Work out the finished part from the listing and answer in its coordinate system (mm). A direction names the side the tool comes from. Round coordinates to 2 decimals unless told otherwise and drop trailing zeros. Order: outer loops, then holes, each group sorted by start corner. A loop starts at its lowest first (then second) coordinate and runs counter-clockwise, first axis right, second up. Notation, with made-up numbers: (-26, 68.25) - (3, 68.25) arc R22 ccw to (3, 80.25) - close; hole circle Ø3 at (88, 35). An arc over 180 degrees is marked (long way). Answer in a Markdown table with one row per item.
from build123d import *

# Parameters (mm, degrees)
ESQUISSE1_W        = 1.5
ESQUISSE1_H        = 20
CHANFREIN1_SIZE    = 0.3
BOSS_EXTRU_1_DEPTH = 2


with BuildPart() as part:
    # Esquisse1 → Base-R_volution (revolve)
    with BuildSketch(Plane(origin=(0, 0, 0), x_dir=(1, 0, 0), z_dir=(0, 1, 0))):
        with Locations((0.75, -10)):
            Rectangle(ESQUISSE1_W, ESQUISSE1_H)
    revolve(axis=Axis((0, 0, 0), (0, 0, 1)))

    # Chanfrein1
    chanfrein1_edges = [part.edges().sort_by_distance(p)[0] for p in [
        (-1.5, 0, 20),
    ]]
    chamfer(chanfrein1_edges, length=CHANFREIN1_SIZE)

    # Esquisse6 → Boss.-Extru.1 (add)
    with BuildSketch(Plane.XY):
        Polygon((2.75, -1.58771324), (2.75, 1.58771324), (0, 3.175426481), (-2.75, 1.58771324), (-2.75, -1.58771324), (0, -3.175426481), align=None)
    extrude(amount=-BOSS_EXTRU_1_DEPTH)

    # Esquisse7 → Enl_vement de mati_re-R_volution1 (revolve, cut)
    with BuildSketch(Plane(origin=(0, 0, 0), x_dir=(1, 0, 0), z_dir=(0, 1, 0)), mode=Mode.PRIVATE) as enl_vement_de_mati_re_r_volution1_sk:
        Polygon((-2.75, 2), (-6.214101615, 2), (-6.214101615, 0), align=None)
    revolve(enl_vement_de_mati_re_r_volution1_sk.sketch.rotate(Axis((0, 0, -6.239446496), (0, 0, 1)), 180), axis=Axis((0, 0, -6.239446496), (0, 0, 1)), mode=Mode.SUBTRACT)  # turned: the seam where the file's is


solid = part.part
1) Find section A-A, the plane z = -0.25. Give the vertices of the cut face in (x, y).
Filled in:
| item | result |
|---|---|
| outline | (-2.75, -1.59) - (0, -3.18) - (2.75, -1.59) - (2.75, 1.59) - (0, 3.18) - (-2.75, 1.59) - close |
2) Find section B-B, the plane z = 8.5. Give the vertices of the cut face in (x, y).
Filled in:
| item | result |
|---|---|
| outline | circle Ø3 at (0, 0) |
3) The mould has two halves that part along Z. Classify faces 1 (the face through (0, 0, 20)), 2 (the face through (-1.394, -2.37, -0.986)), 3 (the face through (2.514, 1.443, -1.914)): released by +Z, released by -Z, zero draft, split by the parting line, or undercut.
Filled in:
| item | result |
|---|---|
| face 1 | released by +Z |
| face 2 | zero draft |
| face 3 | released by -Z |
4) Which of the six approach directions +Z, -Z, +X, -X, +Y, -Y give full straight-line access (tool end or side, diameter ignored) to faces 4 (the face through (-1.5, 0.07, 9.71)), 5 (the face through (-1.36, 2.39, -0.99))?
Filled in:
| item | result |
|---|---|
| face 4 | +Z |
| face 5 | +Z, -Z, -X, +Y |
5) Each of these flat-tipped pins is pushed along its axis until it touches: pin 1 (1.5 mm diameter, centred on y = 2, z = 7, fed in from +X); pin 2 (3 mm diameter, centred on y = 0.5, z = 5.5, fed in from -X); pin 3 (1.5 mm diameter, centred on y = -1.5, z = 10.5, fed in from -X). Where does it stop, or does it pass through?
Filled in:
| item | result |
|---|---|
| pin 1 | stops at x = 0.83 |
| pin 2 | stops at x = -1.5 |
| pin 3 | stops at x = -1.3 |
6) Find the intervals of material crossed by probe 1 along Z at (x, y) = (-1.7, 0.25); probe 2 along X at (y, z) = (-0.75, 10.25); probe 3 along Y at (x, z) = (0, 17.5), in increasing order. Write a range as from..to.
Filled in:
| item | result |
|---|---|
| probe 1 | z = -2..0 |
| probe 2 | x = -1.3..1.3 |
| probe 3 | y = -1.5..1.5 |
